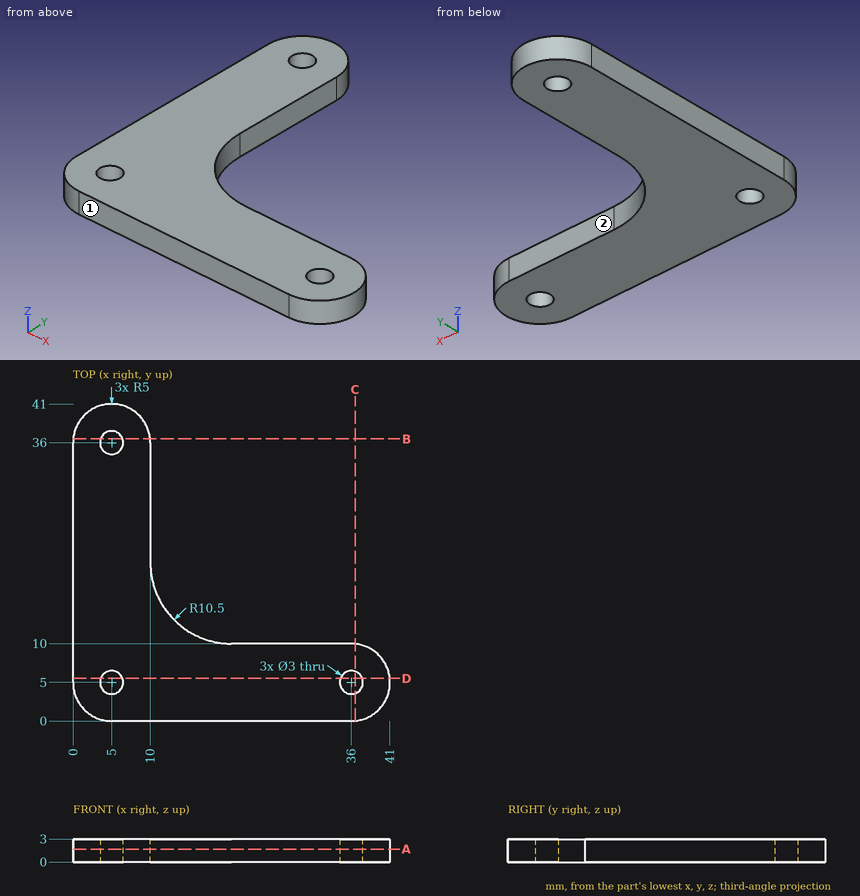
Drawing for the job (mm, zero at the part's lowest x, y, z). A direction names the side the tool comes from. Round coordinates to 2 decimals unless told otherwise and drop trailing zeros. Write each loop counter-clockwise with the first axis right and the second up, starting at its lowest first coordinate (ties: lowest second). Pieces come first, ordered by that corner, then holes. Notation, with made-up numbers: M -19,38 L 21,38 A6 ccw 21,44 Z; hole C 44.5,-2 d11. An arc over 180 degrees is marked long. Answer as a JSON object with one key per item and string values. Group by question number.
(1) Cut at B-B (y = 36.5). Give the cut face in (x, z), and give its area (3 significant figures).
(2) Which spindle directions (+Z, -Z, +X, -X, +Y, -Y) get a long thin tool onto all of the face, cutting with end or side? Do the marked faces 1 and 2. Say none if no direction does.
(3) Cut at A-A (z = 1.7). Give the cut face in (x, y), and give its area (3 significant figures).
(4) Cut at D-D (y = 5.5). Give the cut face in (x, z).
(5) Drill centre lines: L1, parallel to X at y = 22.5, z = 2.05; L2, parallel to X at y = 4.5, z = 2.7. Where is each one in solid material? Low to high.
(6) Flat gauge pins, fed straight in: pin 1 (1.5 mm diameter, centred on x = 28, z = 2, fed in from +Y); pin 2 (0.9 mm diameter, centred on y = 28.5, z = 1, fed in from +X). Where does each tip first touch, or does it go through?
Responses:
{
 "1": {"outline": "M 0.03,0 L 3.59,0 L 3.59,3 L 0.03,3 Z; M 6.41,0 L 9.97,0 L 9.97,3 L 6.41,3 Z", "area": "21.4 mm2"},
 "2": {"face 1": "+Z, -Z, +X, -X, -Y", "face 2": "+Z, -Z, +X, +Y"},
 "3": {"outline": "M 0,5 A5 ccw 5,0 L 36,0 A5 ccw 36,10 L 20.5,10 A10.5 cw 10,20.5 L 10,36 A5 ccw 0,36 Z; hole C 5,5 d3; hole C 5,36 d3; hole C 36,5 d3", "area": "696 mm2"},
 "4": {"outline": "M 0,0 L 3.59,0 L 3.59,3 L 0,3 Z; M 6.41,0 L 34.59,0 L 34.59,3 L 6.41,3 Z; M 37.41,0 L 40.97,0 L 40.97,3 L 37.41,3 Z"},
 "5": {"L1": "x = 0 to 10", "L2": "x = 0.03 to 3.59, 6.41 to 34.59, 37.41 to 40.97"},
 "6": {"pin 1": "stops at y = 10", "pin 2": "stops at x = 10"}
}
